from build123d import *

# Parameters (mm, degrees)
ESQUISSE2_R             = 1.575
ENL_V_MAT_EXTRU_1_DEPTH = 18.205812971
ESQUISSE3_OUTSIDE_W     = 27.986
ESQUISSE3_OUTSIDE_H     = 27.986
ESQUISSE3_OUTSIDE_W_2   = 8
ESQUISSE3_OUTSIDE_H_2   = 20
ENL_V_MAT_EXTRU_2_DEPTH = 18.205812971


with BuildPart() as part:
    # Esquisse1 → Révolution1 (revolve)
    with BuildSketch(Plane.XY, mode=Mode.PRIVATE) as r_volution1_sk:
        Polygon((2.5, 0), (10, 0), (10, 3.2), (4, 3.2), (4, 9.8), (2.5, 9.8), align=None)
    revolve(r_volution1_sk.sketch.rotate(Axis((0, 0, 0), (0, 1, 0)), 90), axis=Axis((0, 0, 0), (0, 1, 0)))

    # Esquisse2 → Enlèv. mat.-Extru.1 (cut, through all)
    with BuildSketch(Plane.XZ):
        with Locations(Location((0, 6.5, 0), (0, 0, 270))):
            Circle(ESQUISSE2_R)
        with Locations(Location((5.629165125, -3.25, 0), (0, 0, 270))):
            Circle(ESQUISSE2_R)
        with Locations(Location((-5.629165125, -3.25, 0), (0, 0, 270))):
            Circle(ESQUISSE2_R)
        with Locations(Location((0, -6.5, 0), (0, 0, 270))):
            Circle(ESQUISSE2_R)
    extrude(amount=-ENL_V_MAT_EXTRU_1_DEPTH, mode=Mode.SUBTRACT)

    # Esquisse3 outside → Enlèv. mat.-Extru.2 (cut, through all)
    with BuildSketch(Plane.XZ):
        Rectangle(ESQUISSE3_OUTSIDE_W, ESQUISSE3_OUTSIDE_H)
        Rectangle(ESQUISSE3_OUTSIDE_W_2, ESQUISSE3_OUTSIDE_H_2, mode=Mode.SUBTRACT)
    extrude(amount=-ENL_V_MAT_EXTRU_2_DEPTH, mode=Mode.SUBTRACT)


solid = part.part
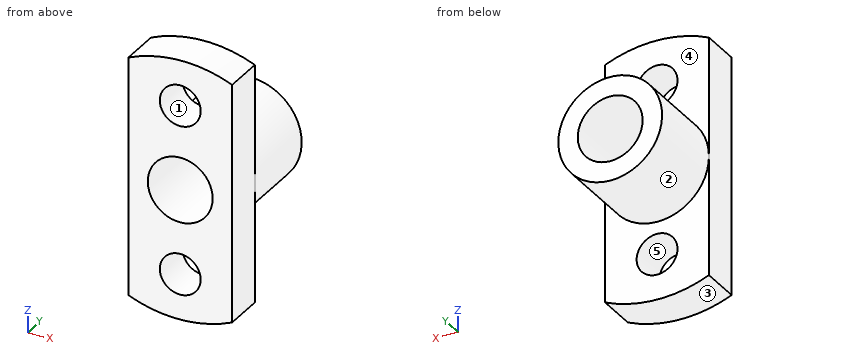
For this review, take the finished solid that the model builds, in its own axes (mm). Face numbers are marked on the shaded views. A direction names the side the tool comes from. Give positions to 0.01 mm unless a question says otherwise; leave off trailing zeros. Write each loop counter-clockwise with the first axis right and the second up, starting at its lowest first coordinate (ties: lowest second). Pieces come first, ordered by that corner, then holes. Notation, with made-up numbers: (23.25, 89.5) -> (73.25, 89.5) arc R19 ccw to (73.25, 118.5) -> close; hole circle Ø1 at (13.25, 14). An arc over 180 degrees is marked (long way). Use CSV: the item, a comma, the result in double quotes.
Q1. Tool access review of the marked faces 1 and 2: name each direction out of +Z, -Z, +X, -X, +Y, -Y from which nothing blocks a thin tool from reaching the whole face with its end or side.
Conclusion:
face 1,"+Y, -Y"
face 2,"+Y"
Q2. For P1, Ø5, axis at y = 8.5, z = -5, coming from the -X side; P2, Ø2, axis at x = -2.5, z = -8, coming from the -Y side, all flat-tipped, find the tip position at first contact; note any pin that passes through.
Conclusion:
P1,"x = -3.12"
P2,"y = 0"
Q3. Take a section at B-B, the plane y = 3. Write out the cut boundary in (x, z) (3 decimals), then the cut area to 3 significant figures.
Conclusion:
outline,"(-4, -9.165) arc R10 ccw to (4, -9.165) -> (4, 9.165) arc R10 ccw to (-4, 9.165) -> close; hole circle Ø5 at (0, 0); hole circle Ø3.15 at (0, -6.5); hole circle Ø3.15 at (0, 6.5)"
area,"120 mm2"
Q4. To check wall thickness, follow probe 1 along X at (y, z) = (3.5, 0); probe 2 along X at (y, z) = (0.9, -6.5) (3 decimals); probe 3 along Z at (x, y) = (0.25, 0.75). State the ranges of each line that lie inside material, in increasing order. Write a range as [from, to].
Conclusion:
probe 1,"[-4, -2.5], [2.5, 4]"
probe 2,"[-4, -1.575], [1.575, 4]"
probe 3,"[-10, -8.06], [-4.94, -2.49], [2.49, 4.94], [8.06, 10]"
Q5. Take a section at A-A, the plane z = 6.5. Write out the cut boundary in (x, y) (3 decimals), then the cut area to 3 significant figures.
Conclusion:
outline,"(-4, 0) -> (-1.575, 0) -> (-1.575, 3.2) -> (-4, 3.2) -> close; (1.575, 0) -> (4, 0) -> (4, 3.2) -> (1.575, 3.2) -> close"
area,"15.5 mm2"
Q6. Take a section at D-D, the plane y = 9. Write out the cut boundary in (x, z).
Conclusion:
outline,"circle Ø8 at (0, 0); hole circle Ø5 at (0, 0)"
Q7. Take a section at C-C, the plane x = 2. Write out the cut boundary in (y, z), then the cut area to 3 significant figures.
Conclusion:
outline,"(0, -9.8) -> (3.2, -9.8) -> (3.2, -3.46) -> (9.8, -3.46) -> (9.8, -1.5) -> (0, -1.5) -> close; (0, 1.5) -> (9.8, 1.5) -> (9.8, 3.46) -> (3.2, 3.46) -> (3.2, 9.8) -> (0, 9.8) -> close"
area,"79.0 mm2"
Q8. Mouldability with a two-part tool opening along Z and no side actions: class the marked faces 3, 4 and 5 as pulls with the +Z half, pulls with the -Z half, needs draft (parallel to the pull), parting line crosses it, or undercut.
Conclusion:
face 3,"pulls with the -Z half"
face 4,"needs draft"
face 5,"undercut"
